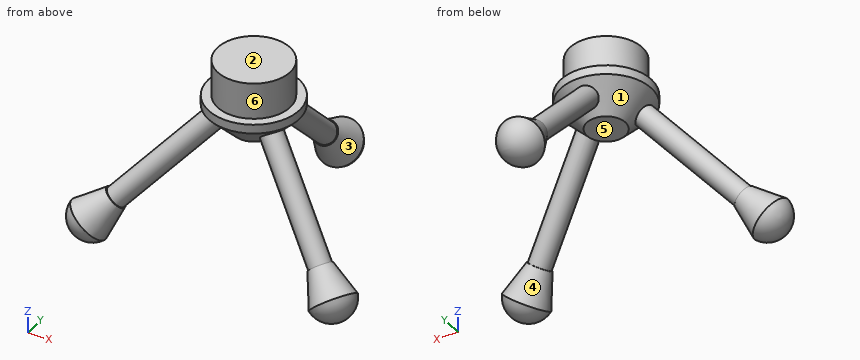
from build123d import *

# Parameters (mm, degrees)
SKETCH1_R                   = 25
BOSS_EXTRUDE1_DEPTH         = 45
CUT_EXTRUDE1_START          = -20
SKETCH2_R                   = 25
SKETCH2_R_2                 = 19.985
CUT_EXTRUDE1_DEPTH          = 20
CHAMFER1_SIZE               = 20
SKETCH3_R                   = 6
BOSS_EXTRUDE2_DEPTH         = 70
CUT_EXTRUDE2_DEPTH          = 70
CUT_EXTRUDE2_DEPTH_BACK     = 70
SKETCH4_W                   = 11.30856595
SKETCH4_H                   = 25.35365412
SKETCH5_R                   = 6.5
BOSS_EXTRUDE3_DEPTH         = 18
BOSS_EXTRUDE3_DRAFT         = -18
CIRPATTERN1_COUNT           = 3
CIRPATTERN1_COPY_1_SKETCH_R = 6.5
CIRPATTERN1_COPY_1_DEPTH    = 18
CIRPATTERN1_COPY_1_DRAFT    = -18
CIRPATTERN1_COPY_2_SKETCH_R = 6.5
CIRPATTERN1_COPY_2_DEPTH    = 18
CIRPATTERN1_COPY_2_DRAFT    = -18


# Read off the part's stored shape, not the designer's step: Dome1
with BuildPart() as part:
    # Sketch1 → Boss-Extrude1 (new body)
    with BuildSketch(Plane.XY):
        with Locations(Location((0, 0, 0), (0, 0, 180))):
            Circle(SKETCH1_R)
    extrude(amount=BOSS_EXTRUDE1_DEPTH)

    # Sketch2 → Cut-Extrude1 (cut)
    with BuildSketch(Plane.XY.offset(45).offset(CUT_EXTRUDE1_START)):
        with Locations(Location((0, 0, 0), (0, 0, 180))):
            Circle(SKETCH2_R)
        Circle(SKETCH2_R_2, mode=Mode.SUBTRACT)
    extrude(amount=CUT_EXTRUDE1_DEPTH, mode=Mode.SUBTRACT)

    # Chamfer1
    chamfer1_edges = [part.edges().sort_by_distance(p)[0] for p in [
        (25, 0, 0),
    ]]
    chamfer(chamfer1_edges, length=CHAMFER1_SIZE)

    # Sketch3 → Boss-Extrude2 (add)
    with BuildSketch(Plane(origin=(0, 0, 0), x_dir=(-1, 0, 0), z_dir=(0, 0.7071067811865475, -0.7071067811865477))):
        with Locations(Location((0, 21.894618235, 0), (0, 0, 291.115116648))):
            Circle(SKETCH3_R)
    boss_extrude2 = extrude(amount=BOSS_EXTRUDE2_DEPTH)

    # Sketch4 → Cut-Extrude2 (cut, two sides: drawn at the far end of the back side and taken through both)
    with BuildSketch(Plane(origin=(0, 0, 0), x_dir=(0, 0, -1), z_dir=(1, 0, 0)).offset(-CUT_EXTRUDE2_DEPTH_BACK)):
        Rectangle(SKETCH4_W, SKETCH4_H)
    extrude(amount=CUT_EXTRUDE2_DEPTH + CUT_EXTRUDE2_DEPTH_BACK, mode=Mode.SUBTRACT)


with BuildPart() as boss_extrude3_tool:
    # Sketch5 → Boss-Extrude3 (with draft: the straight prism first)
    with BuildSketch(Plane(origin=(0, 49.497474683, -49.497474683), x_dir=(1, 0, 0), z_dir=(0, 0.7071067811865476, -0.7071067811865476))):
        with Locations((0, -21.894618235)):
            Circle(SKETCH5_R)
    extrude(amount=BOSS_EXTRUDE3_DEPTH)
    # Boss-Extrude3: the draft: its side faces are tilted about the plane it starts from
    boss_extrude3_sides = [boss_extrude3_tool.faces().sort_by_distance(p)[0] for p in [
        (-6.5, 71.343268739, -40.379602689),
    ]]
    draft(boss_extrude3_sides, Plane(origin=(0, 49.497474683, -49.497474683), x_dir=(1, 0, 0), z_dir=(0, 0.7071067811865476, -0.7071067811865476)), BOSS_EXTRUDE3_DRAFT)


with BuildPart() as part_1:
    add(part.part)

    # Boss-Extrude3: add boss_extrude3_tool
    add(boss_extrude3_tool.part)

    # Dome1 outline → Dome1 (revolve)
    with BuildSketch(Plane(origin=(0, 15.481833025, 15.481833025), x_dir=(1, 0, 0), z_dir=(0, 0.7071067811865476, 0.7071067811865476))):
        with BuildLine():
            Line((0, 88), (12.348554535, 87.999999988))
            ThreePointArc((12.348554535, 87.999999988), (7.944916603, 95.186483631), (0, 98))
            Line((0, 98), (0, 88))
        make_face()
    dome1 = revolve(axis=Axis((0, 15.481833025, 15.481833025), (0, 0.7071067811865476, -0.7071067811865476)))

    # CirPattern1: Boss-Extrude2, Dome1 ×3 about axis
    cirpattern1_axis = Axis((0, 0, 0), (0, 0, 1))
    add([boss_extrude2.rotate(cirpattern1_axis, i * 360 / CIRPATTERN1_COUNT) for i in range(1, CIRPATTERN1_COUNT)])
    add([dome1.rotate(cirpattern1_axis, i * 360 / CIRPATTERN1_COUNT) for i in range(1, CIRPATTERN1_COUNT)])


with BuildPart() as cirpattern1_copy_1_tool:
    # CirPattern1 copy 1 sketch → CirPattern1 copy 1 (with draft: the straight prism first)
    with BuildSketch(Plane(origin=(-42.866070499, -24.748737342, -49.497474683), x_dir=(-0.4999999999999998, 0.8660254037844387, 0), z_dir=(-0.6123724356957946, -0.3535533905932736, -0.7071067811865476))):
        with Locations((0, -21.894618235)):
            Circle(CIRPATTERN1_COPY_1_SKETCH_R)
    extrude(amount=CIRPATTERN1_COPY_1_DEPTH)
    # CirPattern1 copy 1: the draft: its side faces are tilted about the plane it starts from
    cirpattern1_copy_1_sides = [cirpattern1_copy_1_tool.faces().sort_by_distance(p)[0] for p in [
        (-58.535083117, -41.300799494, -40.379602689),
    ]]
    draft(cirpattern1_copy_1_sides, Plane(origin=(-42.866070499, -24.748737342, -49.497474683), x_dir=(-0.4999999999999998, 0.8660254037844387, 0), z_dir=(-0.6123724356957946, -0.3535533905932736, -0.7071067811865476)), CIRPATTERN1_COPY_1_DRAFT)


with BuildPart() as part_2:
    add(part_1.part)

    # CirPattern1 copy 1: add cirpattern1_copy_1_tool
    add(cirpattern1_copy_1_tool.part)


with BuildPart() as cirpattern1_copy_2_tool:
    # CirPattern1 copy 2 sketch → CirPattern1 copy 2 (with draft: the straight prism first)
    with BuildSketch(Plane(origin=(42.866070499, -24.748737342, -49.497474683), x_dir=(-0.5000000000000004, -0.8660254037844384, 0), z_dir=(0.6123724356957944, -0.3535533905932741, -0.7071067811865476))):
        with Locations((0, -21.894618235)):
            Circle(CIRPATTERN1_COPY_2_SKETCH_R)
    extrude(amount=CIRPATTERN1_COPY_2_DEPTH)
    # CirPattern1 copy 2: the draft: its side faces are tilted about the plane it starts from
    cirpattern1_copy_2_sides = [cirpattern1_copy_2_tool.faces().sort_by_distance(p)[0] for p in [
        (65.035083117, -30.042469245, -40.379602689),
    ]]
    draft(cirpattern1_copy_2_sides, Plane(origin=(42.866070499, -24.748737342, -49.497474683), x_dir=(-0.5000000000000004, -0.8660254037844384, 0), z_dir=(0.6123724356957944, -0.3535533905932741, -0.7071067811865476)), CIRPATTERN1_COPY_2_DRAFT)


with BuildPart() as part_3:
    add(part_2.part)

    # CirPattern1 copy 2: add cirpattern1_copy_2_tool
    add(cirpattern1_copy_2_tool.part)


solid = part_3.part
Design review of the part built by this model. Coordinates are the model's own, in mm. Face numbers are marked on the shaded views. A direction names the side the tool comes from. Coordinates: 2 decimals unless noted, no trailing zeros. Order: outer loops, then holes, each group sorted by start corner. A loop starts at its lowest first (then second) coordinate and runs counter-clockwise, first axis right, second up. Notation, with made-up numbers: (-12.75, -8.5) -> (1.25, -8.5) arc R19 ccw to (1.25, -1.5) -> close; hole circle Ø6 at (-25, 84.5). An arc over 180 degrees is marked (long way). Use one line per item in the form item = value. Start each with the question number.
(1) For probe 1 along Y at (x, z) = (5, 10.5); probe 2 along Y at (x, z) = (11.5, 12); probe 3 along Y at (x, z) = (13.5, 36), list the stretches that pass through material, from the lowest coordinate up.
(2) Add section B-B on x = 0. State the section outline as (y, z) points (1 decimal).
(3) Insertion check: pin 1 (17 mm diameter, centred on x = -0.5, y = -0.5, fed in from -Z); pin 2 (2 mm diameter, centred on x = 10, z = 23, fed in from +Y); pin 3 (1 mm diameter, centred on x = 16, y = -5, fed in from -Z). Each pin has a flat end and moves straight along its axis. Give the tip position at first contact, or say it passes through.
(4) For the marked faces 4, 5 and 6, list the 3-axis set-ups (+Z, -Z, +X, -X, +Y, -Y) from which the entire face can be reached by the end or side of a thin tool; tool diameter is ignored.
(5) The part is to be moulded in two halves that separate along X. For the marked faces 1, 2 and 3, say which applies: +X half, -X half, draft (parallel to the pull), parting line (faces both ways), or undercut.
(6) Add section A-A on y = 0. State the section outline as (x, z) points (3 decimals), plus the area to 3 significant figures.
(7) Add section C-C on z = -50. Give the number of separate pieces and of enclosed holes in the cut face, plus the area to 3 significant figures.
Answer block:
q1.probe_1 = -14.67 to 14.67, 15.77 to 25.15
q1.probe_2 = -13.3 to 12.52
q1.probe_3 = -14.74 to 14.74
q2.outline = (-25, 20) -> (-10.7, 5.7) -> (10.7, 5.7) -> (13.7, 8.7) -> (60.7, -38.3) -> (60.4, -38.6) -> (69, -55.5) arc R12.6 ccw to (86.4, -38) -> (69.6, -29.4) -> (69.2, -29.8) -> (22.2, 17.2) -> (25, 20) -> (25, 25) -> (20, 25) -> (20, 45) -> (-20, 45) -> (-20, 25) -> (-25, 25) -> close
q3.pin_1 = 5.65
q3.pin_2 = 23.32
q3.pin_3 = 7.18
q4.face_4 = none
q4.face_5 = -Z, -Y
q4.face_6 = +Z
q5.face_1 = undercut
q5.face_2 = draft
q5.face_3 = parting line
q6.outline = (-25, 20) -> (-10.654, 5.654) -> (10.654, 5.654) -> (25, 20) -> (25, 25) -> (19.985, 25) -> (19.985, 45) -> (-19.985, 45) -> (-19.985, 25) -> (-25, 25) -> close
q6.area = 1,560 mm²
q7.separate_pieces = 3
q7.enclosed_holes = 0
q7.area = 1,120 mm²
